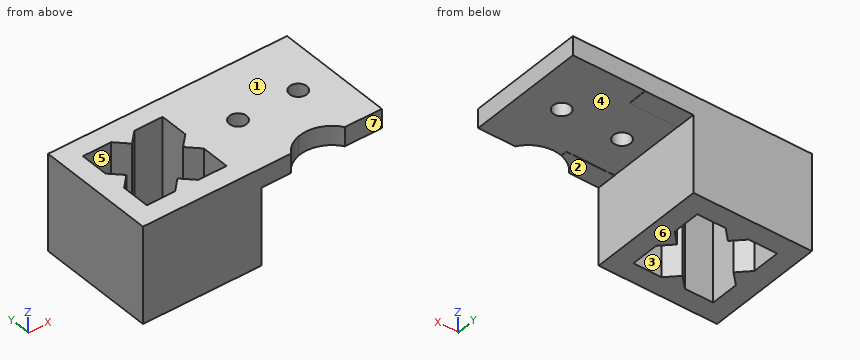
from build123d import *

# Parameters (mm, degrees)
SKETCH1_W            = 31.176
SKETCH1_H            = 31.176
BOSS_EXTRUDE1_DEPTH  = 25.4
BOSS_EXTRUDE2_DEPTH  = 12.7
CUT_EXTRUDE1_DEPTH   = 12.7
SKETCH29_R           = 8.46875
CUT_EXTRUDE10_DEPTH  = 42.089617764
CUT_EXTRUDE11_DEPTH  = 50.166186754
SKETCH30_R           = 2.25
BOSS_EXTRUDE15_DEPTH = 5.019


with BuildPart() as part:
    # Sketch1 → Boss-Extrude1 (new body)
    with BuildSketch(Plane.XY):
        Rectangle(SKETCH1_W, SKETCH1_H)
        Polygon((2.54, -10), (3.048, -10.508), (10.508, -10.508), (10.508, -3.048), (10, -2.54), (7.46, 0), (10, 2.54), (10.508, 3.048), (10.508, 10.508), (3.048, 10.508), (2.54, 10), (0, 7.46), (-2.54, 10), (-3.048, 10.508), (-10.508, 10.508), (-10.508, 3.048), (-10, 2.54), (-7.46, 0), (-10, -2.54), (-10.508, -3.048), (-10.508, -10.508), (-3.048, -10.508), (-2.54, -10), (0, -7.46), align=None, mode=Mode.SUBTRACT)
    extrude(amount=BOSS_EXTRUDE1_DEPTH)

    # Sketch3 → Boss-Extrude2 (add)
    with BuildSketch(Plane(origin=(15.588, 0, 0), x_dir=(0, 0, -1), z_dir=(1, 0, 0))):
        Polygon((-20.381, 10.381), (0, 10.381), (0, 15.588), (-25.4, 15.588), (-25.4, -15.588), (0, -15.588), (0, -10.381), (-20.381, -10.381), align=None)
    extrude(amount=BOSS_EXTRUDE2_DEPTH)

    # Sketch4 → Cut-Extrude1 (cut)
    with BuildSketch(Plane(origin=(0, 0, 20.381), x_dir=(-1, 0, 0), z_dir=(0, 0, -1))):
        with BuildLine():
            ThreePointArc((-24.188, 0), (-21.938, -2.25), (-19.688, 0))
            Line((-19.688, 0), (-24.188, 0))
        make_face()
        with BuildLine():
            Line((-24.188, 0), (-19.688, 0))
            ThreePointArc((-19.688, 0), (-21.938, 2.25), (-24.188, 0))
        make_face()
    extrude(amount=-CUT_EXTRUDE1_DEPTH, mode=Mode.SUBTRACT)

    # Sketch29 → Cut-Extrude10 (cut, through all)
    with BuildSketch(Plane.XY.offset(25.4)):
        with Locations((30.492, -20.220089154)):
            Circle(SKETCH29_R)
    extrude(amount=-CUT_EXTRUDE10_DEPTH, mode=Mode.SUBTRACT)

    # Sketch5 → Cut-Extrude11 (cut, through all)
    with BuildSketch(Plane.XZ.offset(15.588)):
        with BuildLine():
            Line((24.188, 10.32), (28.288, 10.32))
            Line((28.288, 10.32), (28.288, 20.32))
            Line((28.288, 20.32), (15.588, 20.32))
            Line((15.588, 20.32), (15.588, 10.32))
            Line((15.588, 10.32), (19.688, 10.32))
            ThreePointArc((19.688, 10.32), (21.938, 12.57), (24.188, 10.32))
        make_face()
        with BuildLine():
            Line((15.588, 0), (28.288, 0))
            Line((28.288, 0), (28.288, 10.32))
            Line((28.288, 10.32), (24.188, 10.32))
            ThreePointArc((24.188, 10.32), (21.938, 8.07), (19.688, 10.32))
            Line((19.688, 10.32), (15.588, 10.32))
            Line((15.588, 10.32), (15.588, 0))
        make_face()
        with BuildLine():
            ThreePointArc((19.688, 10.32), (21.938, 8.07), (24.188, 10.32))
            Line((24.188, 10.32), (19.688, 10.32))
        make_face()
        with BuildLine():
            Line((19.688, 10.32), (24.188, 10.32))
            ThreePointArc((24.188, 10.32), (21.938, 12.57), (19.688, 10.32))
        make_face()
    extrude(amount=-CUT_EXTRUDE11_DEPTH, mode=Mode.SUBTRACT)

    # Sketch30 → Boss-Extrude15 (add)
    with BuildSketch(Plane.XY.offset(25.4)):
        with BuildLine():
            Line((47.338, 15.588), (28.288, 15.588))
            Line((28.288, 15.588), (28.288, -12.043163658))
            ThreePointArc((28.288, -12.043163658), (33.510098515, -12.307389999), (37.581673944, -15.588))
            Line((37.581673944, -15.588), (47.338, -15.588))
            Line((47.338, -15.588), (47.338, 15.588))
        make_face()
        with Locations((37.813, 0)):
            Circle(SKETCH30_R, mode=Mode.SUBTRACT)
    extrude(amount=-BOSS_EXTRUDE15_DEPTH)


solid = part.part
Input: part model. Units: mm. Frame: model coordinates. Face numbers are marked on the shaded views. A direction names the side the tool comes from. Give positions to 0.01 mm unless a question says otherwise; leave off trailing zeros. Loops run counter-clockwise (first coordinate to the right, second up) from the corner with the lowest first, then second, coordinate; pieces in that order, holes last. Notation, with made-up numbers: M 17.25,78.5 L 67.25,78.5 A18 ccw 67.25,85.5 Z; hole C 19,77.25 d9. An arc over 180 degrees is marked long. Use CSV: the item, a comma, the result in double quotes.
(1) Pin query (flat end, axial travel): P1, Ø15.5, axis at x = 31, y = 4, coming from the -Z side; P2, Ø8, axis at x = 23, z = 11.5, coming from the +Y side; P3, Ø6, axis at y = -4.5, z = 3.5, coming from the +X side. Return the tip coordinate at first contact, or that it passes through.
Outcome:
P1,"stops at z = 20.32"
P2,"passes through"
P3,"stops at x = 15.59"
(2) Section C-C, the plane y = 13. Return loops of the section in (x, z).
Outcome:
outline,"M -15.59,0 L 15.59,0 L 15.59,20.32 L 28.29,20.32 L 28.29,20.38 L 47.34,20.38 L 47.34,25.4 L -15.59,25.4 Z"
(3) Section D-D, the plane y = -1.5. Return loops of the section in (x, z).
Outcome:
outline,"M -15.59,0 L -8.96,0 L -8.96,25.4 L -15.59,25.4 Z; M 8.96,0 L 15.59,0 L 15.59,20.38 L 20.26,20.38 L 20.26,25.4 L 8.96,25.4 Z; M 23.62,20.38 L 36.14,20.38 L 36.14,25.4 L 23.62,25.4 Z; M 39.49,20.38 L 47.34,20.38 L 47.34,25.4 L 39.49,25.4 Z"
(4) Section A-A, the plane y = -6. Return loops of the section in (x, z), plus the area to 3 significant figures.
Outcome:
outline,"M -15.59,0 L -10.51,0 L -10.51,25.4 L -15.59,25.4 Z; M 10.51,0 L 15.59,0 L 15.59,20.38 L 47.34,20.38 L 47.34,25.4 L 10.51,25.4 Z"
area,"417 mm²"
(5) Pull-direction query (Y, two-part tool) for the marked faces 4, 5, 6 and 7; classes: pulls with the +Y half, pulls with the -Y half, needs draft (parallel to the pull), parting line crosses it, or undercut.
Outcome:
face 4,"undercut"
face 5,"undercut"
face 6,"needs draft"
face 7,"pulls with the -Y half"
(6) Set-up query: the marked faces 1, 2 and 3. Return all of +Z, -Z, +X, -X, +Y, -Y with unobstructed straight access to the full face (end or side cutting, diameter ignored); none if empty.
Outcome:
face 1,"+Z, +X, -X, +Y, -Y"
face 2,"-Z, +X, +Y, -Y"
face 3,"+Z, -Z"
(7) Section B-B, the plane z = 23. Return loops of the section in (x, y).
Outcome:
outline,"M -15.59,-15.59 L 23.4,-15.59 A8.47 cw 37.58,-15.59 L 47.34,-15.59 L 47.34,15.59 L -15.59,15.59 Z; hole M -10.51,-10.51 L -3.05,-10.51 L 0,-7.46 L 3.05,-10.51 L 10.51,-10.51 L 10.51,-3.05 L 7.46,0 L 10.51,3.05 L 10.51,10.51 L 3.05,10.51 L 0,7.46 L -3.05,10.51 L -10.51,10.51 L -10.51,3.05 L -7.46,0 L -10.51,-3.05 Z; hole C 21.94,0 d4.5; hole C 37.81,0 d4.5"
(8) Material intervals for L1, parallel to X at y = 5, z = 16.25; L2, parallel to X at y = -10, z = 24.25; L3, parallel to X at y = -12, z = 12.75, sorted ascending. Write a range as [from, to].
Outcome:
L1,"x = [-15.59, -10.51], [10.51, 15.59]"
L2,"x = [-15.59, -10.51], [-2.54, 2.54], [10.51, 47.34]"
L3,"x = [-15.59, 15.59]"
